Drawing for the job (mm, zero at the part's lowest x, y, z). Give positions to 0.01 mm unless a question says otherwise; leave off trailing zeros. Write each loop counter-clockwise with the first axis right and the second up, starting at its lowest first coordinate (ties: lowest second). Pieces come first, ordered by that corner, then holes. Notation, with made-up numbers: M 38.5,41.5 L 94.5,41.5 A16 cw 94.5,67.5 Z; hole C 21.25,4.25 d7. An arc over 180 degrees is marked long. Use CSV: the item, a comma, the result in double quotes. Start each with the question number.
1. Band-saw the part on D-D, the plane x = 13.5. List the corners of the cut face in (y, z), then the cut area to 3 significant figures.
2. Band-saw the part on A-A, the plane x = 47. List the corners of the cut face in (y, z), then the cut area to 3 significant figures.
3. Band-saw the part on C-C, the plane z = 2.75. Count the separate pieces of the cut face and the enclosed holes in it, then the cut area to 3 significant figures.
4. Drill centre lines: line 1 along Y through (x, z) = (47, 2.6); line 2 along Y through (x, z) = (118, 4.45); line 3 along Y through (x, z) = (85, 4.3). Where is each one in solid material? Low to high. Write a range as from..to.
5. Drop flat-ended pins along their axis: pin 1 Ø1.8 at (y, z) = (70, 4) entering from +X; pin 2 Ø3 at (x, z) = (22.5, 4) entering from -Y; pin 3 Ø1.8 at (y, z) = (145.5, 3) entering from -X (3 decimals). Give the stop position or say it passes through.
6. Band-saw the part on B-B, the plane y = 75. List the corners of the cut face in (x, z), then the cut area to 3 significant figures.
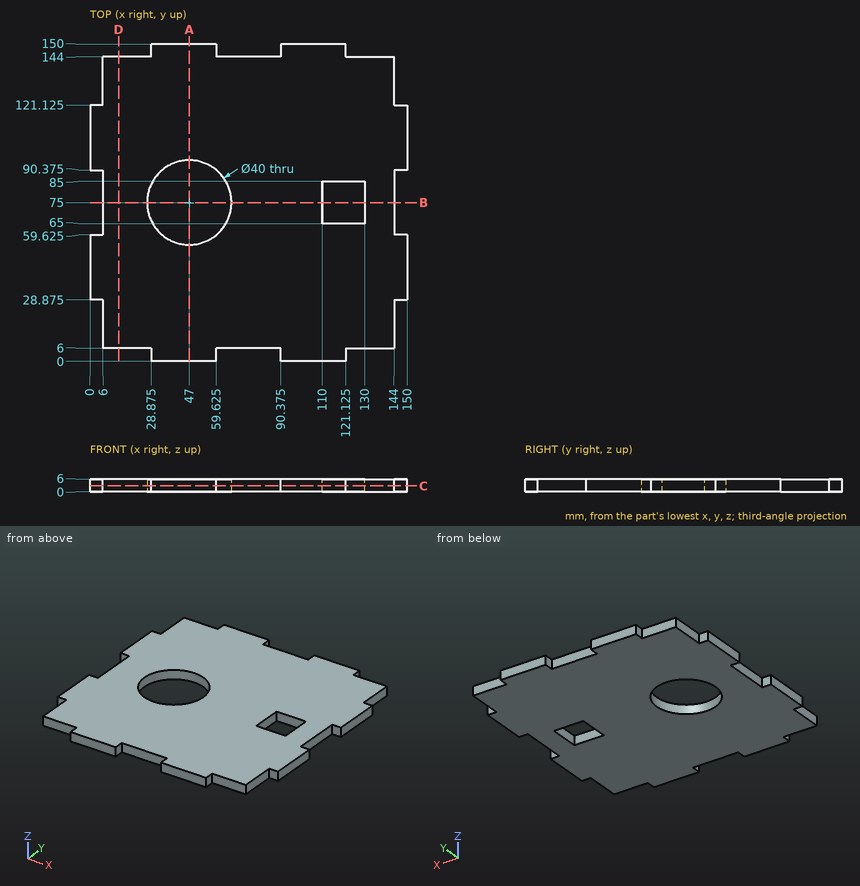
Output:
1,outline,"M 6,0 L 144,0 L 144,6 L 6,6 Z"
1,area,"828 mm²"
2,outline,"M 0,0 L 55,0 L 55,6 L 0,6 Z; M 95,0 L 150,0 L 150,6 L 95,6 Z"
2,area,"660 mm²"
3,separate pieces,"1"
3,enclosed holes,"2"
3,area,"18,900 mm²"
4,line 1,"y = 0..55, 95..150"
4,line 2,"y = 0..65, 85..150"
4,line 3,"y = 6..144"
5,pin 1,"stops at x = 144"
5,pin 2,"stops at y = 6"
5,pin 3,"stops at x = 28.875"
6,outline,"M 6,0 L 27,0 L 27,6 L 6,6 Z; M 67,0 L 110,0 L 110,6 L 67,6 Z; M 130,0 L 144,0 L 144,6 L 130,6 Z"
6,area,"468 mm²"
